from build123d import *

# Parameters (mm, degrees)
F0_R     = 9
F0_R_2   = 3.4
F0_R_3   = 8.5
F0_R_4   = 6.3
F1_DEPTH = 10
F2_DEPTH = 12
F3_DEPTH = 10
F4_DEPTH = 10
F5_DEPTH = 10
F6_DEPTH = 12
F7_DEPTH = 10
F8_DEPTH = 10


# Not quite as in the source:
# - a feature names something its author has since deleted; it is built from what else it names


with BuildPart() as f1:
    # F0 (on Front) → F1 (new body)
    with BuildSketch(Plane.XZ):
        with BuildLine():
            ThreePointArc((57.9036016774, -19.5744080829), (31.1623185662, -12.2328702689), (58.8917768446, -11.9653941064))
            Line((58.8917768446, -11.9653941064), (56.1448434713, 93.81412645))
            ThreePointArc((56.1448434713, 93.81412645), (50.11852804, 107.6101149154), (36.1783402733, 113.2949139834))
            Line((36.1783402733, 113.2949139834), (5.7339191772, 113.3356434663))
            ThreePointArc((5.7339191772, 113.3356434663), (15.6213042052, 109.2285267967), (19.7151895633, 99.3356559948))
            ThreePointArc((19.7151895633, 99.3356559948), (13.3305472737, 87.5880465809), (0, 86.5553348621))
            add(Edge.make_bspline(
                [(27.2971690085, 0), (31.3022406236, 15.2863604375), (39.6477401648, 47.1390527935), (13.5652800367, 73.0692470789), (0, 86.5553348621)],
                knots=[0, 0, 0, 0, 0.4799079546, 1, 1, 1, 1], degree=3))
            Line((27.2971690085, 0), (14.5932951458, -30.2359827701))
            ThreePointArc((14.5932951458, -30.2359827701), (24.2784471497, -53.8293852547), (47.8350505361, -44.0550695737))
            Line((47.8350505361, -44.0550695737), (57.9036016774, -19.5744080829))
        make_face()
        with Locations((31.1880399704, -37.2083886825)):
            Circle(F0_R, mode=Mode.SUBTRACT)
        with Locations((37.6598948849, 72.601060337)):
            Circle(F0_R, mode=Mode.SUBTRACT)
        with Locations((40.1023646421, 101.2938035134)):
            Circle(F0_R_2, mode=Mode.SUBTRACT)
        with BuildLine():
            ThreePointArc((57.9036016774, -19.5744080829), (58.7572249195, -16.863419789), (59.0457295684, -14.0358952114))
            ThreePointArc((59.0457295684, -14.0358952114), (59.0071883365, -12.9977868034), (58.8917768446, -11.9653941064))
            ThreePointArc((58.8917768446, -11.9653941064), (31.1623185662, -12.2328702689), (57.9036016774, -19.5744080829))
        make_face()
        with Locations((45.0457295684, -14.0358952114)):
            Circle(F0_R_3, mode=Mode.SUBTRACT)
        with BuildLine():
            ThreePointArc((19.7151895633, 99.3356559948), (15.6213042052, 109.2285267967), (5.7339191772, 113.3356434663))
            ThreePointArc((5.7339191772, 113.3356434663), (-7.9745381996, 102.2667571151), (0, 86.5553348621))
            ThreePointArc((0, 86.5553348621), (13.3305472737, 87.5880465809), (19.7151895633, 99.3356559948))
        make_face()
        with Locations((5.7151895633, 99.3356559948)):
            Circle(F0_R_3, mode=Mode.SUBTRACT)
        with Locations((37.6598948849, 72.601060337)):
            Circle(F0_R)
        with Locations((37.6598948849, 72.601060337)):
            Circle(F0_R_4, mode=Mode.SUBTRACT)
        with Locations((31.1880399704, -37.2083886825)):
            Circle(F0_R)
        with Locations((31.1880399704, -37.2083886825)):
            Circle(F0_R_4, mode=Mode.SUBTRACT)
        with Locations((45.0457295684, -14.0358952114)):
            Circle(F0_R_3)
        with Locations((5.7151895633, 99.3356559948)):
            Circle(F0_R_3)
        with Locations((31.1880399704, -37.2083886825)):
            Circle(F0_R_4)
        with Locations((37.6598948849, 72.601060337)):
            Circle(F0_R_4)
        with Locations((40.1023646421, 101.2938035134)):
            Circle(F0_R_2)
    extrude(amount=F1_DEPTH)

    # F0 (on Front) → F2 (join)
    with BuildSketch(Plane.XZ):
        with BuildLine():
            ThreePointArc((19.7151895633, 99.3356559948), (15.6213042052, 109.2285267967), (5.7339191772, 113.3356434663))
            ThreePointArc((5.7339191772, 113.3356434663), (-7.9745381996, 102.2667571151), (0, 86.5553348621))
            ThreePointArc((0, 86.5553348621), (13.3305472737, 87.5880465809), (19.7151895633, 99.3356559948))
        make_face()
        with Locations((5.7151895633, 99.3356559948)):
            Circle(F0_R_3, mode=Mode.SUBTRACT)
    extrude(amount=F2_DEPTH)

    # F3 (cut): a face of the model
    f3_faces = [f1.faces().sort_by_distance(p)[0] for p in [
        (5.7151895633, -10, 99.3356559948),
    ]]
    extrude(f3_faces, amount=-F3_DEPTH, mode=Mode.SUBTRACT)

    # F0 (on Front) → F4 (cut)
    with BuildSketch(Plane.XZ):
        with Locations((40.1023646421, 101.2938035134)):
            Circle(F0_R_2)
    extrude(amount=F4_DEPTH, mode=Mode.SUBTRACT)

    # F0 (on Front) → F5 (cut)
    with BuildSketch(Plane.XZ):
        with Locations((37.6598948849, 72.601060337)):
            Circle(F0_R_4)
    extrude(amount=F5_DEPTH, mode=Mode.SUBTRACT)

    # F0 (on Front) → F6 (join)
    with BuildSketch(Plane.XZ):
        with BuildLine():
            ThreePointArc((57.9036016774, -19.5744080829), (58.7572249195, -16.863419789), (59.0457295684, -14.0358952114))
            ThreePointArc((59.0457295684, -14.0358952114), (59.0071883365, -12.9977868034), (58.8917768446, -11.9653941064))
            ThreePointArc((58.8917768446, -11.9653941064), (31.1623185662, -12.2328702689), (57.9036016774, -19.5744080829))
        make_face()
        with Locations((45.0457295684, -14.0358952114)):
            Circle(F0_R_3, mode=Mode.SUBTRACT)
    extrude(amount=F6_DEPTH)

    # F7 (cut): a face of the model
    f7_faces = [f1.faces().sort_by_distance(p)[0] for p in [
        (45.0457295684, -10, -14.0358952114),
    ]]
    extrude(f7_faces, amount=-F7_DEPTH, mode=Mode.SUBTRACT)

    # F0 (on Front) → F8 (cut)
    with BuildSketch(Plane.XZ):
        with Locations((31.1880399704, -37.2083886825)):
            Circle(F0_R_4)
    extrude(amount=F8_DEPTH, mode=Mode.SUBTRACT)


solid = f1.part
The model under review builds one solid part; all positions refer to its coordinate system, in mm. A direction names the side the tool comes from. Give positions to 0.01 mm unless a question says otherwise; leave off trailing zeros. Order: outer loops, then holes, each group sorted by start corner. A loop starts at its lowest first (then second) coordinate and runs counter-clockwise, first axis right, second up. Notation, with made-up numbers: M 43.5,36 L 47.5,36 A15 cw 47.5,54 Z; hole C 68,-12 d9. An arc over 180 degrees is marked long. Answer in a Markdown table with one row per item. Add a question column.
1. For pin 1 Ø3 at (y, z) = (-2.5, 57) entering from +X; pin 2 Ø5 at (x, y) = (25, -4.5) entering from -Z; pin 3 Ø1 at (x, y) = (-1, -3.5) entering from -Z, all flat-tipped, find the tip position at first contact; note any pin that passes through.
2. Machinability: for faces 1 (the cylindrical face through (58.4, -9.53, -18.24)), 2 (the cylindrical face through (43.939, -6.084, -22.464)), 3 (the flat face through (21.034, -4.93, -14.906)), which of the approach directions +Z, -Z, +X, -X, +Y, -Y give a long, thin tool a straight path to every point of the face, cutting with its end or side? Answer none if there is none.
3. Add section B-B on y = -4. Count the separate pieces of the cut face and the enclosed holes in it, plus the area to 3 significant figures.
4. Mouldability with a two-part tool opening along Z and no side actions: class faces 4 (the flat face through (52.799, -4.93, -31.986)), 5 (the cylindrical face through (31.366, -4.93, 72.878)), 6 (the flat face through (40, 0, 30)) as released by +Z, released by -Z, zero draft, split by the parting line, or undercut.
5. To check wall thickness, follow line 1 along Y through (x, z) = (35.5, -26); line 2 along Z through (x, y) = (48.5, -0.75); line 3 along Z through (x, y) = (40.5, -2.5). State the ranges of each line that lie inside material, in increasing order.
6. Add section A-A on x = 46. State the section outline as (y, z) points, plus the area to 3 significant figures.
The answers:
| question | item | result |
|---|---|---|
| 1 | pin 1 | x = 57.14 |
| 1 | pin 2 | z = -54.83 |
| 1 | pin 3 | z = 86.79 |
| 2 | face 1 | -Y |
| 2 | face 2 | +Y, -Y |
| 2 | face 3 | -X, +Y, -Y |
| 3 | separate pieces | 1 |
| 3 | enclosed holes | 5 |
| 3 | area | 5,530 mm2 |
| 4 | face 4 | released by -Z |
| 4 | face 5 | undercut |
| 4 | face 6 | zero draft |
| 5 | line 1 | -10 to 0 |
| 5 | line 2 | -42.44 to -21.8, -6.27 to 109.03 |
| 5 | line 3 | -52.61 to -21.22, -6.85 to 66.98, 78.22 to 97.92, 104.67 to 112.82 |
| 6 | outline | M -12,-28 L -10,-28 L -10,-47.44 L 0,-47.44 L 0,-22.48 L -12,-22.48 Z; M -12,-5.59 L 0,-5.59 L 0,110.7 L -10,110.7 L -10,-0.07 L -12,-0.07 Z |
| 6 | area | 1,430 mm2 |
